Check sheet for the modelled part. Datum: model origin and axes. Units: mm. Face numbers are marked on the shaded views. A direction names the side the tool comes from. Round coordinates to 2 decimals unless told otherwise and drop trailing zeros. Write each loop counter-clockwise with the first axis right and the second up, starting at its lowest first coordinate (ties: lowest second). Pieces come first, ordered by that corner, then holes. Notation, with made-up numbers: (20, 15.5) -> (37, 15.5) arc R21 ccw to (37, 42.5) -> close; hole circle Ø4 at (-18, 77). An arc over 180 degrees is marked (long way). Write item = value, one per line.
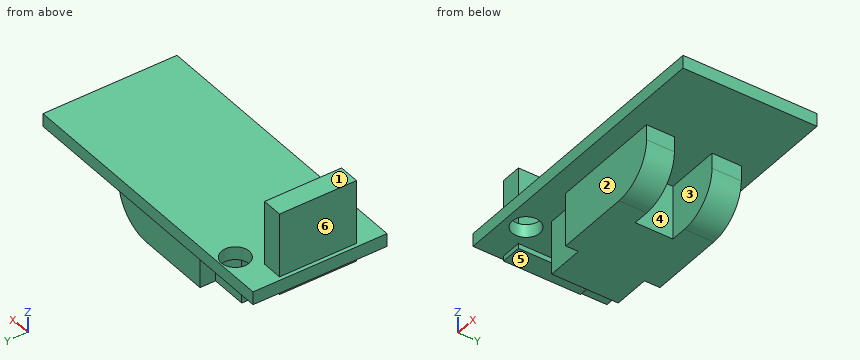
from build123d import *

# Parameters (mm, degrees)
CROQUIS1_W                   = 17.4
CROQUIS1_H                   = 38.1
CROQUIS1_R                   = 1.8
SALIENTE_EXTRUIR1_DEPTH      = 1.7
SALIENTE_EXTRUIR2_DEPTH      = 8.35
SALIENTE_EXTRUIR2_DEPTH_BACK = 2.35
CROQUIS2_W                   = 2.7
CROQUIS2_H                   = 10
SALIENTE_EXTRUIR3_DEPTH      = 7
REDONDEO2_R                  = 5


with BuildPart() as part:
    # Croquis1 → Saliente-Extruir1 (new body)
    with BuildSketch(Plane(origin=(0, 0, 0), x_dir=(0, 1, 0), z_dir=(0, 0, 1))):
        Rectangle(CROQUIS1_W, CROQUIS1_H)
        with Locations(Location((6.7, 13.05, 0), (0, 0, 270))):
            Circle(CROQUIS1_R, mode=Mode.SUBTRACT)
        with Locations(Location((-6.1, 13.05, 0), (0, 0, 270))):
            Circle(CROQUIS1_R, mode=Mode.SUBTRACT)
    extrude(amount=SALIENTE_EXTRUIR1_DEPTH)

    # Croquis2 → Saliente-Extruir2 (add, two sides: drawn at the far end of the back side and taken through both)
    with BuildSketch(Plane.XY.offset(1.7).offset(-SALIENTE_EXTRUIR2_DEPTH_BACK)):
        with Locations((-17.2, -0.1)):
            Rectangle(CROQUIS2_W, CROQUIS2_H)
    extrude(amount=SALIENTE_EXTRUIR2_DEPTH + SALIENTE_EXTRUIR2_DEPTH_BACK)

    # Croquis3 → Saliente-Extruir3 (add)
    with BuildSketch(Plane(origin=(0, 0, 0), x_dir=(1, 0, 0), z_dir=(0, 0, -1))):
        Polygon((-10.690625063, -4.182266508), (-5.944457453, -4.182266508), (-5.944457453, -6.202912125), (8.810954722, -6.202912125), (8.810954722, -2.396579685), (1.715199186, -2.396579685), (1.715199186, 2.490563202), (8.810954722, 2.490563202), (8.810954722, 6.108928608), (-5.850473936, 6.108928608), (-5.850473936, 4.464217059), (-10.690625063, 4.464217059), align=None)
    extrude(amount=SALIENTE_EXTRUIR3_DEPTH)

    # Redondeo2
    redondeo2_edges = [part.edges().sort_by_distance(p)[0] for p in [
        (8.810954722, 4.299745905, -7),
        (8.810954722, -4.299745905, -7),
    ]]
    fillet(redondeo2_edges, radius=REDONDEO2_R)


solid = part.part
(1) Sectioned sample at B-B on y = 5.75. Enter the section's corners in (x, z), then the cut area to 3 significant figures.
Worked answers:
outline = (-19.05, 0) -> (-14.58, 0) -> (-14.58, 1.7) -> (-19.05, 1.7) -> close; (-11.52, 0) -> (-5.94, 0) -> (-5.94, -7) -> (3.81, -7) arc R5 ccw to (8.81, -2) -> (8.81, 0) -> (19.05, 0) -> (19.05, 1.7) -> (-11.52, 1.7) -> close
area = 157 mm²
(2) Sectioned sample at A-A on x = -13.05. Enter the section's corners in (y, z).
Worked answers:
outline = (-8.7, 0) -> (-7.9, 0) -> (-7.9, 1.7) -> (-8.7, 1.7) -> close; (-4.3, 0) -> (4.9, 0) -> (4.9, 1.7) -> (-4.3, 1.7) -> close; (8.5, 0) -> (8.7, 0) -> (8.7, 1.7) -> (8.5, 1.7) -> close
(3) Release check for a two-part mould opening along Y. For the marked faces 1, 2 and 3 record: pulls with the +Y half, pulls with the -Y half, needs draft (parallel to the pull), parting line crosses it, or undercut.
Worked answers:
face_1 = needs draft
face_2 = pulls with the -Y half
face_3 = undercut
(4) Material ranges on L1, parallel to Y at x = -13.05, z = 0.5; L2, parallel to Y at x = 8, z = -2; L3, parallel to Z at x = -12.5, y = -0.75, recorded low to high. Write a range as [from, to].
Worked answers:
L1 = [-8.7, -7.9], [-4.3, 4.9], [8.5, 8.7]
L2 = [-6.11, -2.49], [2.4, 6.2]
L3 = [0, 1.7]
(5) Sectioned sample at D-D on x = -1. Enter the section's corners in (y, z), then the cut area to 3 significant figures.
Worked answers:
outline = (-8.7, 0) -> (-6.11, 0) -> (-6.11, -7) -> (6.2, -7) -> (6.2, 0) -> (8.7, 0) -> (8.7, 1.7) -> (-8.7, 1.7) -> close
area = 116 mm²
(6) Access from +Z, -Z, +X, -X, +Y, -Y to the whole of each face (thin tool, end or side, straight path). Record for the marked faces 4, 5 and 6.
Worked answers:
face_4 = -Z, +X
face_5 = -Z, -X, +Y, -Y
face_6 = +Z, -X, +Y, -Y
(7) Go/stop test with flat-tipped pins: P1, Ø8.5, axis at x = 4.5, y = 2.5, coming from the -Z side; P2, Ø1.6, axis at y = 5, z = -1.5, coming from the +X side; P3, Ø4, axis at x = -14.5, y = -3, coming from the -Z side; P4, Ø1.5, axis at x = -8, z = -2, coming from the -Y side. Record where each tip stops, or that it passes through.
Worked answers:
P1 = -7
P2 = 8.81
P3 = -0.65
P4 = -4.46
(8) Sectioned sample at C-C on y = -3.75. Enter the section's corners in (x, z).
Worked answers:
outline = (-19.05, 0) -> (-18.55, 0) -> (-18.55, -0.65) -> (-15.85, -0.65) -> (-15.85, 0) -> (-10.69, 0) -> (-10.69, -7) -> (3.81, -7) arc R5 ccw to (8.81, -2) -> (8.81, 0) -> (19.05, 0) -> (19.05, 1.7) -> (-15.85, 1.7) -> (-15.85, 10.05) -> (-18.55, 10.05) -> (-18.55, 1.7) -> (-19.05, 1.7) -> close
